```python
from build123d import *

# Parameters (mm, degrees)
SKETCH_1_W          = 2
SKETCH_1_H          = 25
EXTRUDE_1_DEPTH     = 69.5
SKETCH_2_R          = 1.5
SKETCH_2_R_2        = 4
CUT_EXTRUDE_2_DEPTH = 69.5
SKETCH_4_R          = 1.5
CUT_EXTRUDE_3_DEPTH = 10


with BuildPart() as part:
    # 草图1 → 凸台-拉伸1 (new body)
    with BuildSketch(Plane.XY):
        Rectangle(SKETCH_1_W, SKETCH_1_H)
    extrude(amount=EXTRUDE_1_DEPTH)

    # 草图2 → 切除-拉伸2 (cut)
    with BuildSketch(Plane(origin=(1, 0, 0), x_dir=(0, 0, -1), z_dir=(1, 0, 0))):
        with BuildLine():
            Line((0, 12.5), (-12.499054261, 12.5))
            ThreePointArc((-12.499054261, 12.5), (-3.714750597, 8.893031494), (0, 0.153761464))
            Line((0, 0.153761464), (0, 12.5))
        make_face()
        with BuildLine():
            Line((0, -12.5), (0, -0.153761464))
            ThreePointArc((0, -0.153761464), (-3.714750597, -8.893031494), (-12.499054261, -12.5))
            Line((-12.499054261, -12.5), (0, -12.5))
        make_face()
        with Locations(Location((-5.499054261, 0, 0), (0, 0, 90))):
            Circle(SKETCH_2_R)
        with Locations(Location((-12.499054261, 7, 0), (0, 0, 90))):
            Circle(SKETCH_2_R)
        with Locations(Location((-12.499054261, -7, 0), (0, 0, 90))):
            Circle(SKETCH_2_R)
        with Locations(Location((-19.499054261, 0, 0), (0, 0, 90))):
            Circle(SKETCH_2_R)
        with Locations(Location((-12.499054261, 0, 0), (0, 0, 90))):
            Circle(SKETCH_2_R_2)
        with Locations(Location((-31.099054261, 0, 0), (0, 0, 90))):
            Circle(SKETCH_2_R)
    extrude(amount=-CUT_EXTRUDE_2_DEPTH, mode=Mode.SUBTRACT)

    # 草图4 → 切除-拉伸3 (cut)
    with BuildSketch(Plane(origin=(1, 0, 0), x_dir=(0, 0, -1), z_dir=(1, 0, 0))):
        with Locations(Location((-62.6, 0, 0), (0, 0, 90))):
            Circle(SKETCH_4_R)
        with Locations(Location((-56.5, 7, 0), (0, 0, 90))):
            Circle(SKETCH_4_R)
        with Locations(Location((-56.5, -7, 0), (0, 0, 90))):
            Circle(SKETCH_4_R)
    extrude(amount=-CUT_EXTRUDE_3_DEPTH, mode=Mode.SUBTRACT)


solid = part.part
```
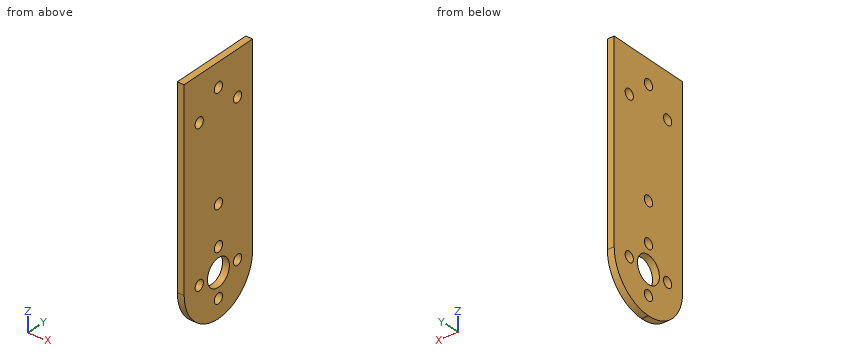
Part model, mm, in its own coordinate system. Round coordinates to 2 decimals unless told otherwise and drop trailing zeros. Loops run counter-clockwise (first coordinate to the right, second up) from the corner with the lowest first, then second, coordinate; pieces in that order, holes last.
Item 1: Cut at D-D, the plane y = 2.75. Give the cut face in (x, z), then the cut area to 3 significant figures.
Item 2: Drill centre lines: line 1 (Y direction, x = -0.65, z = 12.5); line 2 (Z direction, x = -0.55, y = -0.75); line 3 (Z direction, x = -0.05, y = -7). Where is each one in solid material? Low to high.
Item 3: Cut at B-B, the plane y = -7. Give the cut face in (x, z), then the cut area to 3 significant figures.
Item 4: Cut at A-A, the plane z = 56.5. Give the cut face in (x, y), then the cut area to 3 significant figures.
Item 5: Cut at C-C, the plane x = 0.7. State how many separate pieces and enclosed holes the cut face has, then the cut area to 3 significant figures.
A:
1. outline: (-1, 0.31) - (1, 0.31) - (1, 9.59) - (-1, 9.59) - close; (-1, 15.4) - (1, 15.4) - (1, 69.5) - (-1, 69.5) - close
1. area: 127 mm2
2. line 1: y = -12.5 to -8.5, -5.5 to -4, 4 to 5.5, 8.5 to 12.5
2. line 2: z = 0.02 to 4.2, 6.8 to 8.57, 16.43 to 18.2, 20.8 to 29.8, 32.4 to 61.3, 63.9 to 69.5
2. line 3: z = 2.14 to 11, 14 to 55, 58 to 69.5
3. outline: (-1, 2.14) - (1, 2.14) - (1, 11) - (-1, 11) - close; (-1, 14) - (1, 14) - (1, 55) - (-1, 55) - close; (-1, 58) - (1, 58) - (1, 69.5) - (-1, 69.5) - close
3. area: 123 mm2
4. outline: (-1, -12.5) - (1, -12.5) - (1, -8.5) - (-1, -8.5) - close; (-1, -5.5) - (1, -5.5) - (1, 5.5) - (-1, 5.5) - close; (-1, 8.5) - (1, 8.5) - (1, 12.5) - (-1, 12.5) - close
4. area: 38.0 mm2
5. separate pieces: 1
5. enclosed holes: 9
5. area: 1,560 mm2
